Part print with two shaded views. Sizes in mm from the minimum x, y, z corner. Coordinates: 2 decimals unless noted, no trailing zeros. Loops run counter-clockwise (first coordinate to the right, second up) from the corner with the lowest first, then second, coordinate; pieces in that order, holes last.
Item 1: Cut at A-A (y = 29). List the corners of the cut face in (x, z), and give its area (3 significant figures).
Item 2: Cut at B-B (x = 5). List the corners of the cut face in (y, z).
Item 3: Flat gauge pin, fed straight in: pin 1 (3 mm diameter, centred on x = 3.5, y = 2, fed in from +Z). Where does the tip first touch, or does it go through?
Item 4: Cut at C-C (z = 363). List the corners of the cut face in (x, y), and give its area (3 significant figures).
Item 5: Drill centre lines: line 1 along Z through (x, y) = (2, 9.5); line 2 along Y through (x, z) = (2.75, 367.5); line 3 along Y through (x, z) = (5.5, 247). Where is each one in solid material? Low to high.
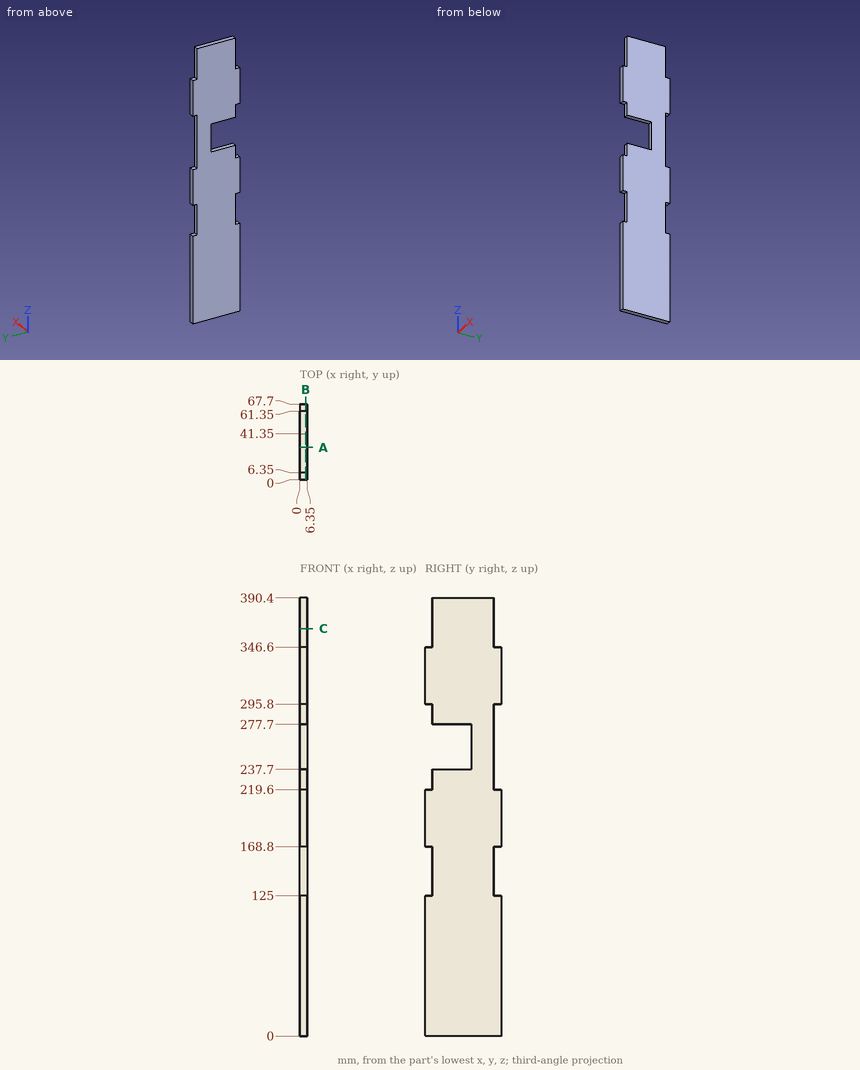
Filled sheet:
1. outline: (0, 0) - (6.35, 0) - (6.35, 237.7) - (0, 237.7) - close; (0, 277.7) - (6.35, 277.7) - (6.35, 390.4) - (0, 390.4) - close
1. area: 2,230 mm2
2. outline: (0, 0) - (67.7, 0) - (67.7, 125) - (61.35, 125) - (61.35, 168.8) - (67.7, 168.8) - (67.7, 219.6) - (61.35, 219.6) - (61.35, 295.8) - (67.7, 295.8) - (67.7, 346.6) - (61.35, 346.6) - (61.35, 390.4) - (6.35, 390.4) - (6.35, 346.6) - (0, 346.6) - (0, 295.8) - (6.35, 295.8) - (6.35, 277.7) - (41.35, 277.7) - (41.35, 237.7) - (6.35, 237.7) - (6.35, 219.6) - (0, 219.6) - (0, 168.8) - (6.35, 168.8) - (6.35, 125) - (0, 125) - close
3. pin 1: stops at z = 346.6
4. outline: (0, 6.35) - (6.35, 6.35) - (6.35, 61.35) - (0, 61.35) - close
4. area: 349 mm2
5. line 1: z = 0 to 237.7, 277.7 to 390.4
5. line 2: y = 6.35 to 61.35
5. line 3: y = 41.35 to 61.35
